from build123d import *

# Parameters (mm, degrees)
CUT_EXTRUDE1_DEPTH  = 33.528
BOSS_EXTRUDE1_DEPTH = 27.178


with BuildPart() as part:
    # Sketch1 → Revolve1 (revolve)
    with BuildSketch(Plane.XY, mode=Mode.PRIVATE) as revolve1_sk:
        with BuildLine():
            Line((528.025465613, 124.987410399), (528.508452089, 123.740780169))
            Line((528.508452089, 123.740780169), (529.612965613, 124.494048207))
            Line((529.612965613, 124.494048207), (535.825761473, 122.563239653))
            Line((535.825761473, 122.563239653), (535.545433806, 121.661224501))
            Line((535.545433806, 121.661224501), (538.723236555, 118.483421752))
            ThreePointArc((538.723236555, 118.483421752), (537.998073772, 110.543513007), (535.87847289, 102.857466948))
            Line((535.87847289, 102.857466948), (530.245653628, 104.608030762))
            Line((530.245653628, 104.608030762), (439.077442195, 132.941226715))
            Line((439.077442195, 132.941226715), (444.657550041, 150.896435606))
            Line((444.657550041, 150.896435606), (528.025465613, 124.987410399))
        make_face()
    revolve(revolve1_sk.sketch.rotate(Axis((439.077442195, 132.941226715, 0), (0.9549466034375443, -0.29677766860580573, 0)), 180), axis=Axis((439.077442195, 132.941226715, 0), (0.9549466034375443, -0.29677766860580573, 0)))

    # Sketch3 → Cut-Extrude1 (cut)
    with BuildSketch(Plane(origin=(438.736808002, -136.350332617, 0), x_dir=(0, 0, -1), z_dir=(0.9549466034375443, -0.2967776686058057, 0))):
        with BuildLine():
            Line((-19.96170913, 257.260152541), (-15.627317141, 257.260152541))
            ThreePointArc((-15.627317141, 257.260152541), (0, 241.632835399), (15.627317141, 257.260152541))
            Line((15.627317141, 257.260152541), (19.96170913, 257.260152541))
            ThreePointArc((19.96170913, 257.260152541), (0, 237.298443411), (-19.96170913, 257.260152541))
        make_face()
    extrude(amount=-CUT_EXTRUDE1_DEPTH, mode=Mode.SUBTRACT)

    # Sketch4 → Boss-Extrude1 (add)
    with BuildSketch(Plane(origin=(435.704852536, -135.408063519, 0), x_dir=(0, 0, 1), z_dir=(-0.9549466034375443, 0.2967776686058057, 0))):
        with BuildLine():
            Line((17.171437949, 254.085152541), (-17.171437949, 254.085152541))
            ThreePointArc((-17.171437949, 254.085152541), (0, 239.797652541), (17.171437949, 254.085152541))
        make_face()
    extrude(amount=BOSS_EXTRUDE1_DEPTH)


solid = part.part
Can you work these out from the model? Positions are in its coordinate system, mm. A direction names the side the tool comes from. Coordinates: 2 decimals unless noted, no trailing zeros. Return JSON: item names as keys, results as strings. Group by question number.
Item 1: I'm going to push flat-ended pins straight in: pin 1 Ø8 at (x, z) = (518, -1.5) entering from +Y; pin 2 Ø6 at (y, z) = (122.5, -1) entering from -X; pin 3 Ø10 at (x, y) = (488.5, 136) entering from +Z. Where does each tip first touch, or does it pass through?
Item 2: If I drill on L1, parallel to Y at x = 490, z = -5.5; L2, parallel to Y at x = 449, z = 1; L3, parallel to Z at x = 457.5, y = 124, over which ranges is the centre line in solid material (lowest first)? Write a range as from..to.
Item 3: Thinking about a two-plate mould opening in Y: for faces 1 (the flat face through (498.317, 111.206, 16.25)), 2 (the cylindrical face through (531.61, 119.81, 11.44)), 3 (the flat face through (439, 132.69, -0.26)), which applies, released by +Y, released by -Y, zero draft, split by the parting line, or undercut?
Item 4: On a 3-axis mill with a long thin cutter (end or side, diameter ignored), from which of +Z, -Z, +X, -X, +Y, -Y can I reach the whole of each face in a straight line? I mean faces 4 (the flat face through (481.32, 102.95, -0.08)), 5 (the flat face through (498.317, 111.206, -16.223)), 6 (the flat face through (507.274, 94.881, -0.08)). Say none if no direction works.
Verdict:
{
 "1": {"pin 1": "stops at y = 129.31", "pin 2": "stops at x = 434.9", "pin 3": "stops at z = 13.97"},
 "2": {"L1": "y = 99.76..135.94", "L2": "y = 110.2..149.52", "L3": "z = -18.55..18.55"},
 "3": {"face 1": "undercut", "face 2": "split by the parting line", "face 3": "released by +Y"},
 "4": {"face 4": "none", "face 5": "-Z", "face 6": "-Y"}
}
